Model file for the job. Use its own axes, mm. A direction names the side the tool comes from. Coordinates: 2 decimals unless noted, no trailing zeros. Order: outer loops, then holes, each group sorted by start corner. A loop starts at its lowest first (then second) coordinate and runs counter-clockwise, first axis right, second up. Notation, with made-up numbers: M -17.5,26 L -9.5,26 A27 ccw -9.5,43 Z; hole C 72,-21 d6. An arc over 180 degrees is marked long. Return JSON: item names as keys, results as strings.
```python
from build123d import *

# Parameters (mm, degrees)
SKETCH1_W           = 30
SKETCH1_H           = 40
BOSS_EXTRUDE1_DEPTH = 15
CUT_EXTRUDE1_DEPTH  = 49
SKETCH3_R           = 1.5
CUT_EXTRUDE2_DEPTH  = 49
SKETCH4_R           = 1.5
BOSS_EXTRUDE2_DEPTH = 25
SKETCH5_W           = 9
SKETCH5_H           = 35
BOSS_EXTRUDE3_DEPTH = 15
SKETCH6_R           = 1.75
BOSS_EXTRUDE4_DEPTH = 15
SKETCH7_W           = 15
SKETCH7_H           = 40
BOSS_EXTRUDE6_DEPTH = 30
CUT_EXTRUDE3_DEPTH  = 59
SKETCH10_R          = 1.5
CUT_EXTRUDE4_DEPTH  = 59


with BuildPart() as part:
    # Sketch1 → Boss-Extrude1 (new body)
    with BuildSketch(Plane.XY):
        with Locations((15, 20)):
            Rectangle(SKETCH1_W, SKETCH1_H)
    extrude(amount=BOSS_EXTRUDE1_DEPTH)

    # Sketch2 → Cut-Extrude1 (cut)
    with BuildSketch(Plane(origin=(0, 40, 0), x_dir=(1, 0, 0), z_dir=(0, 1, 0))):
        with BuildLine():
            Line((7.5, -15), (22.5, -15))
            ThreePointArc((22.5, -15), (15, -7.5), (7.5, -15))
        make_face()
    extrude(amount=-CUT_EXTRUDE1_DEPTH, mode=Mode.SUBTRACT)

    # Sketch3 → Cut-Extrude2 (cut)
    with BuildSketch(Plane.XY.offset(15)):
        with Locations((3, 34)):
            Circle(SKETCH3_R)
        with Locations((3, 6)):
            Circle(SKETCH3_R)
        with Locations((27, 34)):
            Circle(SKETCH3_R)
        with Locations((27, 6)):
            Circle(SKETCH3_R)
    extrude(amount=-CUT_EXTRUDE2_DEPTH, mode=Mode.SUBTRACT)

    # Sketch4 → Boss-Extrude2 (add)
    with BuildSketch(Plane(origin=(30, 0, 0), x_dir=(0, 0, -1), z_dir=(1, 0, 0))):
        with Locations(Location((-3, 34, 0), (0, 0, 180))):
            Circle(SKETCH4_R)
        with Locations(Location((-3, 6, 0), (0, 0, 180))):
            Circle(SKETCH4_R)
    extrude(amount=BOSS_EXTRUDE2_DEPTH)

    # Sketch5 → Boss-Extrude3 (add)
    with BuildSketch(Plane(origin=(55, 0, 0), x_dir=(0, 0, -1), z_dir=(1, 0, 0))):
        with Locations((-4.5, 20)):
            Rectangle(SKETCH5_W, SKETCH5_H)
    extrude(amount=BOSS_EXTRUDE3_DEPTH)

    # Sketch6 → Boss-Extrude4 (add)
    with BuildSketch(Plane(origin=(70, 0, 0), x_dir=(0, 0, -1), z_dir=(1, 0, 0))):
        with Locations(Location((-5.5, 33, 0), (0, 0, 180))):
            Circle(SKETCH6_R)
        with Locations(Location((-5.5, 6.887482194, 0), (0, 0, 180))):
            Circle(SKETCH6_R)
    extrude(amount=BOSS_EXTRUDE4_DEPTH)

    # Sketch7 → Boss-Extrude6 (add)
    with BuildSketch(Plane(origin=(85, 0, 0), x_dir=(0, 0, -1), z_dir=(1, 0, 0))):
        with Locations((-7.5, 20)):
            Rectangle(SKETCH7_W, SKETCH7_H)
    extrude(amount=BOSS_EXTRUDE6_DEPTH)

    # Sketch9 → Cut-Extrude3 (cut)
    with BuildSketch(Plane(origin=(0, 40, 0), x_dir=(1, 0, 0), z_dir=(0, 1, 0))):
        with BuildLine():
            Line((92.5, -15), (107.5, -15))
            ThreePointArc((107.5, -15), (100, -7.5), (92.5, -15))
        make_face()
    extrude(amount=-CUT_EXTRUDE3_DEPTH, mode=Mode.SUBTRACT)

    # Sketch10 → Cut-Extrude4 (cut)
    with BuildSketch(Plane.XY.offset(15)):
        with Locations((88, 34)):
            Circle(SKETCH10_R)
        with Locations((112, 34)):
            Circle(SKETCH10_R)
        with Locations((112, 6)):
            Circle(SKETCH10_R)
        with Locations((88, 6)):
            Circle(SKETCH10_R)
    extrude(amount=-CUT_EXTRUDE4_DEPTH, mode=Mode.SUBTRACT)


solid = part.part
```
Item 1: Saw through at A-A (x = 27). Write the cut outline in (y, z), and give its area (3 significant figures).
Check result:
{"outline": "M 0,0 L 4.5,0 L 4.5,15 L 0,15 Z; M 7.5,0 L 32.5,0 L 32.5,15 L 7.5,15 Z; M 35.5,0 L 40,0 L 40,15 L 35.5,15 Z", "area": "510 mm2"}
Item 2: Pull direction X, two halves, no side cores. Call faces 1 (the flat face through (15, 20, 0)), 2 (the flat face through (0, 20, 7)), 3 (the cylindrical face through (89.43, 6.45, 7.6)), 4 (the cylindrical face through (42.325, 35.464, 2.675)): +X half, -X half, draft (parallel to the pull), parting line (faces both ways), or undercut.
Check result:
{"face 1": "draft", "face 2": "-X half", "face 3": "undercut", "face 4": "undercut"}
Item 3: 3-axis set-ups, long thin cutter, end or side, ignore diameter. For faces 5 (the flat face through (62, 2.5, 5)), 6 (the flat face through (62, 37.5, 5)), 7 (the cylindrical face through (77.395, 31.265, 5.272)): which of +Z, -Z, +X, -X, +Y, -Y reach the whole face in a straight line?
Check result:
{"face 5": "+Z, -Z, -Y", "face 6": "+Z, -Z, +Y", "face 7": "none"}
Item 4: Saw through at C-C (y = 19). Write the cut outline in (x, z).
Check result:
{"outline": "M 0,0 L 30,0 L 30,15 L 22.5,15 A7.5 cw 7.5,15 L 0,15 Z; M 55,0 L 70,0 L 70,9 L 55,9 Z; M 85,0 L 115,0 L 115,15 L 107.5,15 A7.5 cw 92.5,15 L 85,15 Z"}
Item 5: Wall check: line 1 (Y direction, x = 88, z = 10); line 2 (X direction, y = 19.5, z = 3); line 3 (X direction, y = 32, z = 6.5). Give the ranges that are in metal, low to high.
Check result:
{"line 1": "y = 0 to 4.5, 7.5 to 32.5, 35.5 to 40", "line 2": "x = 0 to 30, 55 to 70, 85 to 115", "line 3": "x = 0 to 30, 55 to 115"}
Item 6: Saw through at B-B (z = 5.5). Count the separate pieces of the cut face and the enclosed holes in it, and give its area (3 significant figures).
Check result:
{"separate pieces": "2", "enclosed holes": "9", "area": "2,970 mm2"}
Item 7: Drop flat-ended pins along their axis: pin 1 Ø1.8 at (x, y) = (112, 6) entering from -Z; pin 2 Ø2 at (x, y) = (80.5, 33) entering from +Z; pin 3 Ø4.5 at (x, y) = (64.5, 11.5) entering from +Z; pin 4 Ø1.5 at (x, z) = (51, 5) entering from +Y. Give the stop position or say it passes through.
Check result:
{"pin 1": "passes through", "pin 2": "stops at z = 7.25", "pin 3": "stops at z = 9", "pin 4": "stops at y = 34.83"}
